from build123d import *

# Parameters (mm, degrees)
F1_R     = 2.75
F1_R_2   = 1.5
F2_DEPTH = 2
F3_START = 1.5
F3_DEPTH = 0.5
F4_START = 2
F4_DEPTH = 26
F5_SIZE2 = 1.25
F5_SIZE  = 1.25
F6_R     = 0.25


# Not quite as in the source:
# - a feature names something its author has since deleted; it is built from what else it names


with BuildPart() as f2:
    # F1 (on Top) → F2 (new body)
    with BuildSketch(Plane.XY):
        Circle(F1_R)
        Circle(F1_R_2, mode=Mode.SUBTRACT)
        Circle(F1_R_2)
        Polygon((-0.5773502692, -1), (-1.1547005384, 0), (-0.5773502692, 1), (0.5773502692, 1), (1.1547005384, 0), (0.5773502692, -1), align=None, mode=Mode.SUBTRACT)
    extrude(amount=F2_DEPTH)

    # F1 (on Top) → F3 (join)
    with BuildSketch(Plane.XY.offset(F3_START)):
        Polygon((-0.5773502692, 1), (-1.1547005384, 0), (-0.5773502692, -1), (0.5773502692, -1), (1.1547005384, 0), (0.5773502692, 1), align=None)
    extrude(amount=F3_DEPTH)

    # F1 (on Top) → F4 (join)
    with BuildSketch(Plane.XY.offset(F4_START)):
        Circle(F1_R_2)
        Polygon((-0.5773502692, -1), (-1.1547005384, 0), (-0.5773502692, 1), (0.5773502692, 1), (1.1547005384, 0), (0.5773502692, -1), align=None, mode=Mode.SUBTRACT)
        Polygon((-0.5773502692, 1), (-1.1547005384, 0), (-0.5773502692, -1), (0.5773502692, -1), (1.1547005384, 0), (0.5773502692, 1), align=None)
    extrude(amount=F4_DEPTH)

    # F5
    f5_edges = [f2.edges().sort_by_distance(p)[0] for p in [
        (-2.75, 0, 0),
    ]]
    chamfer(f5_edges, length=F5_SIZE, length2=F5_SIZE2)

    # F6
    f6_edges = [f2.edges().sort_by_distance(p)[0] for p in [
        (-2.75, 0, 2),
        (-1.5, 0, 2),
        (-1.5, 0, 0),
        (-2.75, 0, 1.25),
    ]]
    fillet(f6_edges, radius=F6_R)


solid = f2.part
Input: part model. Units: mm. Frame: model coordinates. A direction names the side the tool comes from. Coordinates: 2 decimals unless noted, no trailing zeros. Order: outer loops, then holes, each group sorted by start corner. A loop starts at its lowest first (then second) coordinate and runs counter-clockwise, first axis right, second up.
1. Ray query, line 1 along Z through (x, y) = (0.1, 0.65); line 2 along Y through (x, z) = (-0.55, 24.5); line 3 along X through (y, z) = (1.3, 23). Return the intervals inside material, ascending.
Checked values:
line 1: z = 1.5 to 28
line 2: y = -1.4 to 1.4
line 3: x = -0.75 to 0.75
2. Draft query along Y for faces 3 (the flat face through (1, 2, 2)), 4 (the cylindrical face through (-1.5, 0.07, 14.94)), 5 (the flat face through (0, 1, 1)). Return one class per face: +Y half, -Y half, draft (parallel to the pull), parting line (faces both ways), or undercut.
Checked values:
face 3: draft
face 4: parting line
face 5: undercut
3. Access query for faces 1 (the flat face through (0, 0, 1.5)), 2 (the cylindrical face through (-0.596, -2.685, 1.549)). Directions: +Z, -Z, +X, -X, +Y, -Y. A direction counts if a zero-diameter tool reaches every point of the face in a straight line with its end or side. Return the directions, or none.
Checked values:
face 1: -Z
face 2: +Z, -Z
4. Contact query for flat-ended pins moving along their axis: P1, Ø2, axis at y = -1, z = 22, coming from the +X side; P2, Ø1, axis at y = -1, z = 24.5, coming from the -X side; P3, Ø1, axis at x = 1.5, y = 2, coming from the +Z side. Output: stop coordinate, or through.
Checked values:
P1: stops at x = 1.5
P2: stops at x = -1.41
P3: stops at z = 2
5. Cut plane A-A, the plane z = 8.5. Return loops of the section in (x, y).
Checked values:
outline: circle Ø3 at (0, 0)
